Work out the finished part from the listing and answer in its coordinate system (mm). A direction names the side the tool comes from. Round coordinates to 2 decimals unless told otherwise and drop trailing zeros. Loops run counter-clockwise (first coordinate to the right, second up) from the corner with the lowest first, then second, coordinate; pieces in that order, holes last. Notation, with made-up numbers: M 54.25,88.5 L 74.25,88.5 A27 ccw 74.25,119.5 Z; hole C 16.25,11.25 d1. An arc over 180 degrees is marked long. One line per item, written item: value.
```python
from build123d import *

# Parameters (mm, degrees)
SKETCH052_R          = 5.08
POCKET_DEPTH         = 161.926
POCKET013_DEPTH      = 1086.426433
POCKET013_DEPTH_BACK = 1378.526433
POLARPATTERN_COUNT   = 8
SKETCH080_R          = 15.875
POCKET014_DEPTH      = 224.597427


with BuildPart() as part:
    # Sketch003 → Revolution (revolve)
    with BuildSketch(Plane.XZ):
        with BuildLine():
            ThreePointArc((38.1, 152.4), (11.159232, 141.240768), (0, 114.3))
            Line((0, 114.3), (2.683626, 108.544946))
            Line((2.683626, 108.544946), (2.683626, 62.824946))
            Line((2.683626, 62.824946), (5.367252, 57.069891))
            Line((5.367252, 57.069891), (5.367252, 0))
            Line((5.367252, 0), (8.574284, 0))
            Line((8.574284, 58.565355), (8.574284, 0))
            Line((5.890658, 64.320409), (8.574284, 58.565355))
            Line((5.890658, 110.040409), (5.890658, 64.320409))
            Line((3.207032, 115.795464), (5.890658, 110.040409))
            ThreePointArc((38.1, 149.225), (13.938806, 139.518889), (3.207032, 115.795464))
            Line((285.75, 149.225), (38.1, 149.225))
            ThreePointArc((285.75, 149.225), (290.240128, 151.084872), (292.1, 155.575))
            Line((292.1, 161.925), (292.1, 155.575))
            Line((288.925, 161.925), (292.1, 161.925))
            Line((288.925, 155.575), (288.925, 161.925))
            ThreePointArc((285.75, 152.4), (287.995064, 153.329936), (288.925, 155.575))
            Line((38.1, 152.4), (285.75, 152.4))
        make_face()
    revolve(axis=Axis((0, 0, 0), (1, 0, 0)))

    # Sketch052 → Pocket (cut, through all)
    with BuildSketch(Plane.XZ):
        with Locations((101.6, 0)):
            Circle(SKETCH052_R)
    extrude(amount=POCKET_DEPTH, mode=Mode.SUBTRACT)

    # Sketch004 → Pocket013 (cut, two sides)
    with BuildSketch(Plane.YZ) as pocket013_sk:
        with BuildLine():
            Line((158.813657, 31.59), (155.285786, 26.310168))
            ThreePointArc((155.285786, 26.310168), (154.825454, 25.231136), (154.788371, 24.058601))
            ThreePointArc((154.788371, -24.058601), (156.646916, 0), (154.788371, 24.058601))
            ThreePointArc((154.788371, -24.058601), (154.825454, -25.231136), (155.285786, -26.310168))
            Line((158.813657, -31.59), (155.285786, -26.310168))
            ThreePointArc((158.813657, -31.59), (161.925, 0), (158.813657, 31.59))
        make_face()
    pocket013 = extrude(amount=-POCKET013_DEPTH, mode=Mode.SUBTRACT) + extrude(pocket013_sk.sketch, amount=POCKET013_DEPTH_BACK, mode=Mode.SUBTRACT)

    # PolarPattern: Pocket013 ×8 about axis
    polarpattern_axis = Axis((0, 0, 0), (1, 0, 0))
    for i in range(1, POLARPATTERN_COUNT):
        add(pocket013.rotate(polarpattern_axis, i * 360 / POLARPATTERN_COUNT), mode=Mode.SUBTRACT)

    # Sketch080 (on DatumPlane) → Pocket014 (cut, through all)
    with BuildSketch(Plane(origin=(0, 0, 0), x_dir=(1, 0, 0), z_dir=(0, -0.707107, -0.707107))):
        with Locations((68.58, 0)):
            Circle(SKETCH080_R)
    extrude(amount=POCKET014_DEPTH, mode=Mode.SUBTRACT)


solid = part.part
```
1) The mould has two halves that part along Y. Classify faces 5 (the face through (290.53, 111, 110.53)), 6 (the face through (290.53, -111, -110.53)), 7 (the face through (5.237, 34.896, -45.51)): +Y half, -Y half, draft (parallel to the pull), parting line (faces both ways), or undercut.
Check values:
face 5: +Y half
face 6: -Y half
face 7: undercut
2) For faces 1 (the face through (8.574, -1, -1)), 2 (the face through (106.445, -150.747, 1.526)), 3 (the face through (290.535, 62.377, 149.428)), 4 (the face through (163.659, 135.205, 70.323)), determine the directions among +Z, -Z, +X, -X, +Y, -Y from which every point of the face is accessible in a straight line to the end or side of a thin tool.
Check values:
face 1: +X
face 2: -Y
face 3: +Z, +X, -X, +Y
face 4: -X
3) Find section A-A (x = 143). Give the vertices of the cut face in (y, z) (3 decimals).
Check values:
outline: C 0,0 d304.8; hole C 0,0 d298.45
4) Find the intervals of material crossed by probe 1 along Y at (x, z) = (218, 0) (3 decimals); probe 2 along X at (y, z) = (-9.5, 77.5); probe 3 along Y at (x, z) = (63, 77), in increasing order. Write a range as from..to.
Check values:
probe 1: -152.4..-149.225, 149.225..152.4
probe 2: 2.68..5.89
probe 3: -131.52..-127.82, 127.82..131.52
5) Each of these flat-tipped pins is pushed along its axis until it touches: pin 1 (3 mm diameter, centred on x = 204.5, z = -52.5, fed in from +Y); pin 2 (1.5 mm diameter, centred on x = 169, z = -89, fed in from +Y); pin 3 (2 mm diameter, centred on y = -1, z = -40.5, fed in from +X). Where does it stop, or does it pass through?
Check values:
pin 1: y = 143.61
pin 2: y = 124.25
pin 3: x = 8.57
